Autodesk Inventor part; units mm, degrees
ref_plane "Work Plane1" through (31.995545, 31.552354, -2) normal (-0.4998287, 0.0130885, 0.8660254) x (-0.0261769, -0.9996573, 0)
ref_plane "YZ Plane" through (0, 0, 0) normal (1, 0, 0) x (0, 1, 0)
ref_plane "XZ Plane" through (0, 0, 0) normal (0, 1, 0) x (-1, 0, 0)
sketch "Sketch1" plane through (0, 0, 0) normal (0, 0, 1) x (1, 0, 0)
  line L0 (-19, 46.892654) -> (19, 46.892654)
  line L1 (33.99486, 31.5) -> (32.345147, -31.5)
  arc A0 (33.99486, 31.5) -> (19, 46.892654) centre (19, 31.892654) ccw
  line L2 (-19, 44.892654) -> (19, 44.892654)
  arc A1 (31.995545, 31.552354) -> (19, 44.892654) centre (19, 31.892654) ccw
  line L3 (31.995545, 31.552354) -> (30.344461, -31.5)
  line L4 (-19, 46.892654) -> (-19, 44.892654)
  line L5 (30.344461, -31.5) -> (32.345147, -31.5)
  point P0 (0, 0)
  point P1 (33.170003, 0)
  point P2 (0, 46.892654)
  dimension "d0" = 88.5
  dimension "d1" = 15
  dimension "d2" = 38
  dimension "d3" = 63
  dimension "d4" = 2
extrude "Extrusion1" add sketch "Sketch1" against normal blind 11
sketch "Sketch3" plane through (-19, 44.892654, 0) normal (0, -1, 0) x (1, 0, 0)
  line L0 (0, 0) -> (13, 0)
  line L1 (13, 0) -> (13, -14.7)
  line L2 (13, -14.7) -> (0, -14.7)
  line L3 (0, -14.7) -> (0, 0)
  line L4 (0, 0) -> (38, 0)
  line L5 (0, 0) -> (0, -11)
  point P0 (19, 0)
  dimension "d7" = 13
  dimension "d8" = 14.7
extrude "Extrusion2" [suppressed]
extrude "Extrusion3" [suppressed]
sketch "Sketch5" plane through (-19, 42.692654, 0) normal (0, -1, 0) x (1, 0, 0)
  line L0 (0, 0) -> (6.5, 0) construction
  line L1 (6.5, 0) -> (6.5, -4.77) construction
  line L2 (6.5, -4.77) -> (0, -4.77) construction
  line L3 (0, -4.77) -> (0, 0) construction
  line L4 (13, 0) -> (0, 0) construction
  line L5 (0, 0) -> (0, -14.7) construction
  circle A0 centre (6.5, -4.77) radius 1.8
  circle A1 centre (6.5, -4.77) radius 3.5
  point P0 (19, 0)
  dimension "d15" = 4.77
  dimension "d16" = 6.5
  dimension "d17" = 3.6
  dimension "d18" = 7
extrude "Extrusion7" [suppressed]
extrude "Extrusion8" [suppressed]
sketch "Sketch7" plane through (-19, 42.692654, 0) normal (-1, 0, 0) x (0, 0, 1)
  line L0 (-6.57, 3) -> (-2.97, 3)
  line L1 (-6.57, 5.2) -> (-2.97, 5.2)
  line L2 (-6.57, 5.2) -> (-12.7, 5.2)
  line L3 (-12.7, 5.2) -> (-12.7, 1.7)
  line L4 (-12.7, 1.7) -> (-6.57, 1.7)
  line L5 (-6.57, 1.7) -> (-6.57, 5.2)
  line L6 (0, 5.2) -> (-14.7, 5.2)
  line L7 (-14.7, 5.2) -> (-14.7, 0)
  point P0 (0, -42.692654)
  point P1 (-12.7, 3.45)
  dimension "d31" = 3.5
  dimension "d32" = 2
extrude "Extrusion9" [suppressed]
sketch "Sketch8" plane through (-19, 46.892654, 0) normal (0, 1, 0) x (1, 0, 0)
  line L0 (38, 11) -> (0, 11)
  line L1 (13, 11) -> (18, 11)
  line L2 (18, 11) -> (18, 6.57)
  line L3 (18, 6.57) -> (13, 6.57)
  line L4 (13, 6.57) -> (13, 11)
  line L5 (13, 6.57) -> (6.5, 6.57)
  point P0 (19, 0)
  dimension "d35" = 5
extrude "Extrusion10" [suppressed]
chamfer "Chamfer1" [suppressed]
sketch "Sketch9" plane through (31.995545, 31.552354, -11) normal (-0.9996573, 0.0261769, 0) x (0, 0, 1)
  line L0 (9, 0) -> (9, -63.073968)
  line L1 (11, -63.073968) -> (0, -63.073968)
  line L2 (11, 0) -> (0, 0)
  line L3 (11, 0) -> (11, -63.073968)
  point P0 (11, -32.379087)
  dimension "d41" = 2
ref_plane "Work Plane1" through (31.995545, 31.552354, -2) normal (-0.4998287, 0.0130885, 0.8660254) x (-0.0261769, -0.9996573, 0)
sketch "Sketch10" plane through (31.995545, 31.552354, -2) normal (-0.4998287, 0.0130885, 0.8660254) x (-0.0261769, -0.9996573, 0)
  line L0 (47.073968, -32) -> (63.073968, -32)
  line L1 (63.073968, -32) -> (63.073968, 0)
  line L2 (63.073968, 0) -> (47.073968, 0)
  line L3 (47.073968, 0) -> (47.073968, -32)
  line L4 (63.073968, 1) -> (63.073968, -4.5)
  line L5 (0, 1) -> (63.073968, 1)
  line L6 (0, 1) -> (0, -4.5)
  line L7 (63.073968, -4.5) -> (0, -4.5)
  line L8 (63.073968, 1) -> (63.073968, -4.5)
  line L9 (0, 0) -> (63.073968, 0)
  line L10 (0.073968, -21.6) -> (47.073968, -21.6)
  line L11 (47.073968, -21.6) -> (47.073968, -10.4)
  line L12 (47.073968, -10.4) -> (0.073968, -10.4)
  line L13 (0.073968, -10.4) -> (0.073968, -21.6)
  point P0 (32.379087, -25.984171)
  point P1 (47.073968, -16)
  point P2 (47.073968, -16)
  point P3 (47.073968, -4.5)
  dimension "d43" = 32
  dimension "d44" = 16
  dimension "d45" = 11.2
  dimension "d46" = 47
extrude "Extrusion11" add sketch "Sketch10" against normal blind 4 contours L3 L7 L1 L0 | L10 L13 L12 L3 | L7 L3 L2 L1
sketch "Sketch12" plane through (23.759029, -15.32207, -10.664102) normal (0.8657286, -0.0226699, 0.5) x (0.4998287, -0.0130885, -0.8660254)
  line L0 (-4, 0) -> (-4, 47)
  line L1 (-4, 0) -> (0, 0)
  line L2 (0, 47) -> (0, 0)
  line L3 (-4, 47) -> (0, 47)
  line L4 (-4, 38.228587) -> (-4, 47)
  point P0 (-21.311369, 14.69488)
extrude "Extrusion13" add sketch "Sketch12" along normal up to surface surface through (33.99486, 31.5, 0) normal (0.9996573, -0.0261769, 0)
sketch "Sketch15" plane through (2.641145, -30.774563, -18) normal (-0.0261769, -0.9996573, 0) x (0.8657286, -0.0226699, 0.5)
  line L0 (29.690599, -4) -> (27.5, -7.794229)
  line L1 (27.5, -7.794229) -> (20.928203, -4)
  line L2 (10.4, -4) -> (29.690599, -4)
  line L3 (21.446961, 8.402201) -> (33, 1.732051)
  line L4 (21.446961, 8.402201) -> (15.946961, -1.124078)
  line L5 (27.5, -7.794229) -> (15.946961, -1.124078)
  line L6 (33, 1.732051) -> (27.5, -7.794229)
  point P0 (6.015829, 17.311369)
extrude "Extrusion16" add sketch "Sketch15" against normal up to surface (63 mm away) contours L0 L1 L2
sketch "Sketch14" plane through (31.995545, 31.552354, -2) normal (-0.4998287, 0.0130885, 0.8660254) x (0.8657286, -0.0226699, 0.5)
  line L0 (-29, -49.573968) -> (-3, -49.573968) construction
  line L1 (-3, -49.573968) -> (-3, -60.573968) construction
  line L2 (-3, -60.573968) -> (-29, -60.573968) construction
  line L3 (-29, -60.573968) -> (-29, -49.573968) construction
  line L4 (-21.6, -0.073968) -> (-21.6, -47.073968) construction
  line L5 (-21.6, -47.073968) -> (-32, -47.073968) construction
  line L6 (-32, -47.073968) -> (-32, -63.073968) construction
  line L7 (-32, -63.073968) -> (0, -63.073968) construction
  line L8 (0, -0.073968) -> (0, -63.073968) construction
  circle A0 centre (-29, -49.573968) radius 0.95
  circle A1 centre (-29, -60.573968) radius 0.95
  circle A2 centre (-3, -60.573968) radius 0.95
  circle A3 centre (-3, -49.573968) radius 0.95
  line L9 (0, -0.073968) -> (-21.6, -0.073968)
  point P0 (-25.984171, -32.379087)
  point P1 (-16, -63.073968)
  point P2 (-16, -60.573968)
  point P3 (-29, -55.073968)
  point P4 (-32, -55.073968)
  dimension "d58" = 26
  dimension "d59" = 11
  dimension "d60" = 1.9
extrude "Extrusion15" cut sketch "Sketch14" against normal blind 20
sketch "Sketch17" plane through (12.063554, -15.015813, -12.8) normal (-0.8657286, 0.0226699, -0.5) x (-0.4998287, 0.0130885, 0.8660254)
  line L0 (0, 47) -> (0, 0)
  line L1 (0, 30) -> (7.92723, 47)
  line L2 (7.92723, 47) -> (0, 47)
  point P0 (17.311369, 14.69488)
  dimension "d67" = 17
  dimension "d68" = 25
extrude "Extrusion17" add sketch "Sketch17" against normal up to surface (11.2 mm away)
sketch "Sketch19" plane through (12.848862, 14.973907, -12.8) normal (-0.4640615, -0.4106113, 0.7848856) x (0.8657286, -0.0226699, 0.5)
  line L0 (11.2, 0) -> (11.2, 18.757425)
  line L1 (0, 18.757425) -> (11.2, 18.757425)
  line L2 (0, 0) -> (0, 18.757425)
  line L3 (11.2, 0) -> (0, 0)
  line L4 (1, 1) -> (1, 17.757425)
  line L5 (1, 17.757425) -> (10.2, 17.757425)
  line L6 (10.2, 17.757425) -> (10.2, 1)
  line L7 (10.2, 1) -> (1, 1)
  line L8 (1, 1) -> (1, 0)
  line L9 (10.2, 1) -> (10.2, 0)
  point P0 (-4.384171, -6.555048)
  dimension "d71" = 1
  dimension "d72" = 9.2
extrude "Extrusion18" add sketch "Sketch19" along normal blind 2 contours L3 L9 L6 L5 L4 L8 L2 L1 L0
sketch "Sketch20" plane through (13.714591, 14.951237, -12.3) normal (0.1875123, -0.9115286, -0.3659982) x (0.8657286, -0.0226699, 0.5)
  line L0 (10.2, 0) -> (9.2, 0)
  line L1 (10.2, 0) -> (10.2, 2)
  line L2 (9.2, 2) -> (10.2, 2)
  line L3 (9.2, 0) -> (9.2, 2)
  line L4 (0, 0) -> (-1, 0)
  line L5 (0, 0) -> (0, 2)
  line L6 (-1, 2) -> (0, 2)
  line L7 (-1, 0) -> (-1, 2)
  point P0 (-5.384171, 22.157652)
extrude "Extrusion19" add sketch "Sketch20" along normal up to surface surface through (14.907242, 0.281044, -11.389944) normal (-0.4998287, 0.0130885, 0.8660254)
sketch "Sketch21" plane through (-19, 46.892654, 0) normal (0, 1, 0) x (1, 0, 0)
  line L0 (52.99486, 0) -> (52.99486, 11)
  circle A0 centre (23.89486, 4.77) radius 1.8
  line L1 (38, 0) -> (0, 0)
  line L2 (38, 0) -> (0, 0)
  line L3 (38, 0) -> (38, 11)
  line L4 (0, 11) -> (38, 11)
  line L5 (0, 0) -> (0, 11)
  line L6 (18.89486, 0) -> (18.89486, 11)
  point P0 (19, 0)
  dimension "d77" = 29.1
  dimension "d78" = 3.6
  dimension "d79" = 4.77
  dimension "d80" = 5
extrude "Extrusion20" cut sketch "Sketch21" against normal up to surface (2 mm away) contours A0 | L1 L5 L4 L6
sketch "Sketch24" plane through (31.993609, 31.478411, -2) normal (0.0261769, 0.9996573, 0) x (0.9996573, -0.0261769, 0)
  line L0 (-12.970279, -1.665183) -> (-9.006664, 5.2)
  line L1 (-1.775352, 1.025) -> (-3.4208, 1.975)
  line L2 (-1.775352, 1.025) -> (-3.4208, 1.975)
  line L3 (-27.712813, 16) -> (0, 0)
  line L4 (0, 0) -> (-9.006664, 5.2)
  line L5 (0, 0) -> (-12.970279, -1.665183)
  line L6 (-9.87269, 5.7) -> (-17.840123, 10.3)
  line L7 (-12.970279, -1.665183) -> (-13.876587, -3.234954)
  line L8 (-13.876587, -3.234954) -> (-9.006664, 5.2)
  line L9 (-17.840123, 10.3) -> (-18.706149, 10.8)
  line L10 (-9.006664, 5.2) -> (-9.87269, 5.7)
  line L11 (-18.706149, 10.8) -> (-27.712813, 16)
  point P0 (-31.158637, -2)
  point P1 (-21.487547, 18.030192)
  point P2 (-22.943031, 19.251489)
  point P3 (-21.487547, 18.030192)
  point P4 (-22.943031, 19.251489)
  point P5 (0, 0)
  point P6 (-1.775352, 1.025)
  point P7 (-3.4208, 1.975)
  point P8 (-9.006664, 5.2)
extrude "Extrusion22" add sketch "Sketch24" against normal up to surface surface through (15.010195, 22.574698, -4.997638) normal (-0.4640615, -0.4106113, 0.7848856)
equation "\"d68\" = zangle"
equation "\"yangle\" = 30deg"
equation "\"zangle\" = 25deg"
equation "\"d42\" = yangle"
properties part number "3DOCameraMount_3DPrint"
Geometry: final body of the model. Coordinates: model frame, mm. A direction names the side the tool comes from. Give positions to 0.01 mm unless a question says otherwise; leave off trailing zeros. Loops run counter-clockwise (first coordinate to the right, second up) from the corner with the lowest first, then second, coordinate; pieces in that order, holes last. Notation, with made-up numbers: (-31, -20.75) -> (-23, -20.75) arc R5 cw to (-23, -16.75) -> close; hole circle Ø2 at (-6.75, 49). An arc over 180 degrees is marked (long way). Use one line per item in the form item = value.
Item 1: Pin query (flat end, axial travel): P1, Ø8, axis at y = 10.5, z = -6, coming from the +X side; P2, Ø1.5, axis at x = 11.5, z = -13.5, coming from the +Y side; P3, Ø9, axis at x = 11, z = -7.5, coming from the -Y side. Return the tip coordinate at first contact, or that it passes through.
A:
P1 = 33.55
P2 = -14.98
P3 = 12.34
Item 2: Draft query along Z for faces 3 (the face through (13.65, 31.54, -2.4)), 4 (the face through (29.9, 42.2, -5.4)), 5 (the face through (7.04, -28.75, -17.77)). Return one class per face: pulls with the +Z half, pulls with the -Z half, needs draft (parallel to the pull), parting line crosses it, or undercut.
A:
face_3 = pulls with the +Z half
face_4 = needs draft
face_5 = undercut
Item 3: Section query D-D on y = 17.5. Output: boundary loops of the cut face in (x, z).
A:
outline = (11.23, -9.89) -> (14.92, -16.26) -> (24.04, -11) -> (33.63, -11) -> (33.63, 0) -> (31.63, 0) -> (31.63, -2) -> (25.83, -1.26) -> (20.02, -4.69) -> (21.11, -6.59) -> (13.19, -11.28) -> (12.09, -9.38) -> close
Item 4: Line query: probe 1 along X at (y, z) = (45.65, -4.77); probe 2 along Z at (x, y) = (32.5, 21.5); probe 3 along X at (y, z) = (45.55, -4.77). Output: solid intervals per line, ascending.
A:
probe_1 = -0.11 to 3.09, 6.69 to 24.98
probe_2 = -11 to 0
probe_3 = -0.11 to 3.09, 6.69 to 25.2
Item 5: Section query B-B on y = -21. Output: boundary loops of the cut face in (x, z).
A:
outline = (2.9, -18) -> (4.9, -21.46) -> (23.03, -11) -> (32.62, -11) -> (32.62, 0) -> (30.62, 0) -> (30.62, -2) -> close
Item 6: Section query C-C on z = -14. Output: boundary loops of the cut face in (x, y), and give its area (3 significant figures).
A:
outline = (9.57, -30.96) -> (17.56, -31.17) -> (19.21, 31.81) -> (13.99, 31.95) -> (12.76, -15.03) -> (9.99, -14.96) -> close
area = 374 mm^2
Item 7: Section query A-A on x = 20. Output: boundary loops of the cut face in (y, z), and give its area (3 significant figures).
A:
outline = (-31.23, -12.59) -> (31.79, -13.55) -> (31.79, -0.46) -> (25.57, -0.48) -> (17.57, -4.66) -> (22.91, -4.42) -> (14.79, -8.67) -> (-31.23, -7.97) -> close; (44.85, -11) -> (46.86, -11) -> (46.86, 0) -> (44.85, 0) -> close
area = 410 mm^2
Item 8: Access query for faces 1 (the face through (7.328, -17.757, -17.769)), 2 (the face through (9, 44.893, -5)). Directions: +Z, -Z, +X, -X, +Y, -Y. A direction counts if a zero-diameter tool reaches every point of the face in a straight line with its end or side. Return the directions, or none.
A:
face_1 = none
face_2 = +Z, -Z, -X
